The model under review builds one solid part; all positions refer to its coordinate system, in mm. Coordinates: 2 decimals unless noted, no trailing zeros. Loops run counter-clockwise (first coordinate to the right, second up) from the corner with the lowest first, then second, coordinate; pieces in that order, holes last. Notation, with made-up numbers: M 72,-20.5 L 101,-20.5 A21 ccw 101,12.5 Z; hole C -26.5,62.25 d8. An arc over 180 degrees is marked long. Return JSON: item names as keys, results as strings.
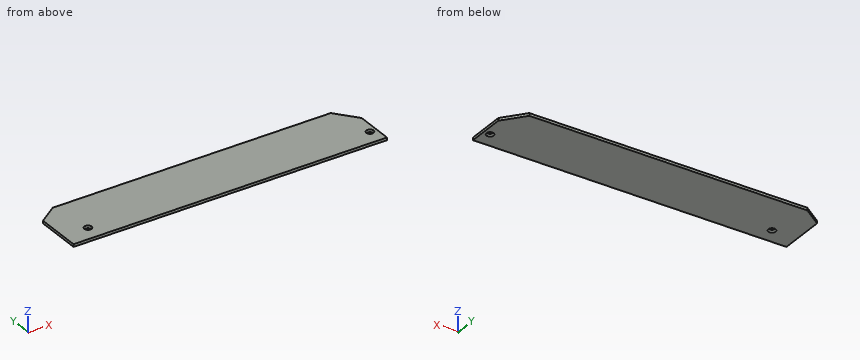
```python
from build123d import *

# Parameters (mm, degrees)
LOW_SIDE_SHIELD_WITH_ENDS_CHAMFERED_PROF_R = 2.75
LOW_SIDE_SHIELD_WITH_ENDS_CHAMFERED_DEPTH  = 2


with BuildPart() as part:
    # Low side shield with ends chamfered profile → Low side shield with ends chamfered (new body)
    with BuildSketch(Plane.XY):
        Polygon((-136, 7), (103, 7), (103, 36), (90, 52), (-122, 52), (-136, 42), align=None)
        with Locations((-117, 19)):
            Circle(LOW_SIDE_SHIELD_WITH_ENDS_CHAMFERED_PROF_R, mode=Mode.SUBTRACT)
        with Locations((98, 19)):
            Circle(LOW_SIDE_SHIELD_WITH_ENDS_CHAMFERED_PROF_R, mode=Mode.SUBTRACT)
    extrude(amount=LOW_SIDE_SHIELD_WITH_ENDS_CHAMFERED_DEPTH)


solid = part.part
```
1. Add section B-B on z = 0.75. Give the boundary of the cut face in (x, y).
Check values:
{"outline": "M -136,7 L 103,7 L 103,36 L 90,52 L -122,52 L -136,42 Z; hole C -117,19 d5.5; hole C 98,19 d5.5"}
2. Add section C-C on x = 98. Give the boundary of the cut face in (y, z), plus the area to 3 significant figures.
Check values:
{"outline": "M 7,0 L 16.25,0 L 16.25,2 L 7,2 Z; M 21.75,0 L 42.15,0 L 42.15,2 L 21.75,2 Z", "area": "59.3 mm²"}
3. Add section A-A on x = -117. Give the boundary of the cut face in (y, z), plus the area to 3 significant figures.
Check values:
{"outline": "M 7,0 L 16.25,0 L 16.25,2 L 7,2 Z; M 21.75,0 L 52,0 L 52,2 L 21.75,2 Z", "area": "79.0 mm²"}
4. To check wall thickness, follow line 1 (X direction, y = 18, z = 0.8); line 2 (Y direction, x = -117, z = 0.8); line 3 (Y direction, x = 98, z = 0.8). State the ranges of each line that lie inside material, in increasing order.
Check values:
{"line 1": "-136 to -119.56, -114.44 to 95.44, 100.56 to 103", "line 2": "7 to 16.25, 21.75 to 52", "line 3": "7 to 16.25, 21.75 to 42.15"}
